from build123d import *

# Parameters (mm, degrees)
SKETCH1_W           = 86
SKETCH1_H           = 57
BOSS_EXTRUDE1_DEPTH = 10
SKETCH2_R           = 2
CUT_EXTRUDE1_DEPTH  = 67.213669284
SKETCH4_W           = 96
SKETCH4_H           = 66
SKETCH4_W_2         = 82
SKETCH4_H_2         = 52
BOSS_EXTRUDE2_DEPTH = 2
SKETCH6_W           = 54
SKETCH6_H           = 5
CUT_EXTRUDE2_DEPTH  = 5
SKETCH7_W           = 43
SKETCH7_H           = 5
CUT_EXTRUDE3_DEPTH  = 5
CHAMFER1_SIZE       = 2
CHAMFER2_SIZE       = 1
CHAMFER3_SIZE       = 1
CHAMFER4_SIZE       = 1
SKETCH9_R           = 3.75
CUT_EXTRUDE4_DEPTH  = 2.7
SKETCH10_W          = 65
SKETCH10_H          = 6
CUT_EXTRUDE5_DEPTH  = 4.5
SKETCH11_W          = 14
SKETCH11_H          = 6
CUT_EXTRUDE6_DEPTH  = 4.5


with BuildPart() as part:
    # Sketch1 → Boss-Extrude1 (new body)
    with BuildSketch(Plane(origin=(0, 0, 0), x_dir=(1, 0, 0), z_dir=(0, 1, 0))):
        with BuildLine():
            Line((48, -33), (48, 33))
            Line((48, 33), (-33, 33))
            Line((-33, 33), (-33, 39.5))
            ThreePointArc((-33, 39.5), (-38, 44.5), (-43, 39.5))
            Line((-43, 39.5), (-43, 33))
            Line((-43, 33), (-48, 33))
            Line((-48, 33), (-48, -33))
            Line((-48, -33), (-38, -33))
            Line((-38, -33), (-38, -39.5))
            ThreePointArc((-38, -39.5), (-33, -44.5), (-28, -39.5))
            Line((-28, -39.5), (-28, -33))
            Line((-28, -33), (28, -33))
            Line((28, -33), (28, -39.5))
            ThreePointArc((28, -39.5), (33, -44.5), (38, -39.5))
            Line((38, -39.5), (38, -33))
            Line((38, -33), (48, -33))
        make_face()
        Rectangle(SKETCH1_W, SKETCH1_H, mode=Mode.SUBTRACT)
    extrude(amount=BOSS_EXTRUDE1_DEPTH)

    # Sketch2 → Cut-Extrude1 (cut, through all)
    with BuildSketch(Plane(origin=(0, 10, 0), x_dir=(1, 0, 0), z_dir=(0, 1, 0))):
        with Locations(Location((-38, 39.5, 0), (0, 0, 270))):
            Circle(SKETCH2_R)
        with Locations(Location((33, -39.5, 0), (0, 0, 270))):
            Circle(SKETCH2_R)
        with Locations(Location((-33, -39.5, 0), (0, 0, 270))):
            Circle(SKETCH2_R)
    extrude(amount=-CUT_EXTRUDE1_DEPTH, mode=Mode.SUBTRACT)

    # Sketch4 → Boss-Extrude2 (add)
    with BuildSketch(Plane(origin=(0, 10, 0), x_dir=(1, 0, 0), z_dir=(0, 1, 0))):
        Rectangle(SKETCH4_W, SKETCH4_H)
        Rectangle(SKETCH4_W_2, SKETCH4_H_2, mode=Mode.SUBTRACT)
    extrude(amount=BOSS_EXTRUDE2_DEPTH)

    # Sketch6 → Cut-Extrude2 (cut)
    with BuildSketch(Plane.ZY.offset(48)):
        with Locations((0, 2.5)):
            Rectangle(SKETCH6_W, SKETCH6_H)
    extrude(amount=-CUT_EXTRUDE2_DEPTH, mode=Mode.SUBTRACT)

    # Sketch7 → Cut-Extrude3 (cut)
    with BuildSketch(Plane(origin=(48, 0, 0), x_dir=(0, 0, -1), z_dir=(1, 0, 0))):
        with Locations((1.5, 2.5)):
            Rectangle(SKETCH7_W, SKETCH7_H)
    extrude(amount=-CUT_EXTRUDE3_DEPTH, mode=Mode.SUBTRACT)

    # Chamfer1
    chamfer1_edges = [part.edges().sort_by_distance(p)[0] for p in [
        (-41, 12, 0),
        (0, 12, 26),
        (41, 12, 0),
        (0, 12, -26),
    ]]
    chamfer(chamfer1_edges, length=CHAMFER1_SIZE - 0.0001)  # a hair under: the kernel refuses the full size

    # Chamfer2
    chamfer2_edges = [part.edges().sort_by_distance(p)[0] for p in [
        (-48, 12, 0),
        (0, 12, 33),
        (48, 12, 0),
        (0, 12, -33),
    ]]
    chamfer(chamfer2_edges, length=CHAMFER2_SIZE)

    # Chamfer3
    chamfer3_edges = [part.edges().sort_by_distance(p)[0] for p in [
        (-48, 5.5, -33),
    ]]
    chamfer(chamfer3_edges, length=CHAMFER3_SIZE)

    # Chamfer4
    chamfer4_edges = [part.edges().sort_by_distance(p)[0] for p in [
        (48, 5.5, 33),
        (-48, 5.5, 33),
        (48, 5.5, -33),
    ]]
    chamfer(chamfer4_edges, length=CHAMFER4_SIZE)

    # Sketch9 → Cut-Extrude4 (cut)
    with BuildSketch(Plane(origin=(0, 10, 0), x_dir=(1, 0, 0), z_dir=(0, 1, 0))):
        with Locations(Location((-38, 39.5, 0), (0, 0, 270))):
            Circle(SKETCH9_R)
        with Locations(Location((-33, -39.5, 0), (0, 0, 270))):
            Circle(SKETCH9_R)
        with Locations(Location((33, -39.5, 0), (0, 0, 270))):
            Circle(SKETCH9_R)
    extrude(amount=-CUT_EXTRUDE4_DEPTH, mode=Mode.SUBTRACT)

    # Sketch10 → Cut-Extrude5 (cut)
    with BuildSketch(Plane(origin=(0, 0, -33), x_dir=(-1, 0, 0), z_dir=(0, 0, -1))):
        with Locations((0.5, 3)):
            Rectangle(SKETCH10_W, SKETCH10_H)
    extrude(amount=-CUT_EXTRUDE5_DEPTH, mode=Mode.SUBTRACT)

    # Sketch11 → Cut-Extrude6 (cut)
    with BuildSketch(Plane.XY.offset(33)):
        with Locations((-21, 3)):
            Rectangle(SKETCH11_W, SKETCH11_H)
    extrude(amount=-CUT_EXTRUDE6_DEPTH, mode=Mode.SUBTRACT)


solid = part.part
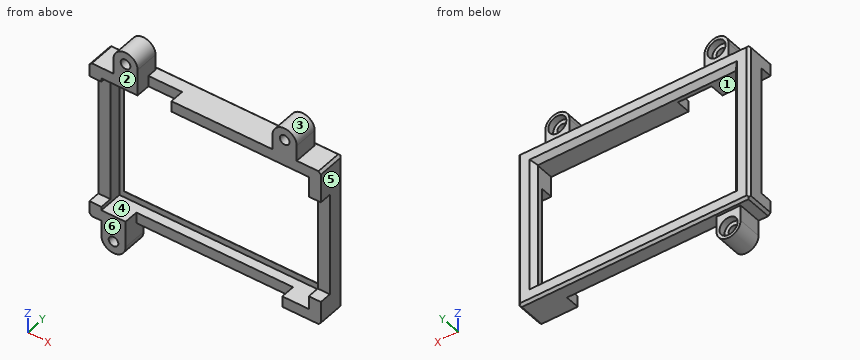
Read the model definition and answer for the solid it produces. Units are mm, in the model's axes. Face numbers are marked on the shaded views. A direction names the side the tool comes from. Round coordinates to 2 decimals unless told otherwise and drop trailing zeros.
1) Straight lines are drawn through the part: L1, parallel to X at y = 5.5, z = 39.5; L2, parallel to X at y = 8.7, z = 39.5; L3, parallel to X at y = 5, z = 35.5. For each, find the intervals that lie inside material, in ascending order.
2) Flat-ended cylindrical pins translate along their axes: pin 1 (8.5 mm diameter, centred on x = -33, z = 39.5, fed in from +Y); pin 2 (5.5 mm diameter, centred on x = 44.5, y = 2.5, fed in from +Z); pin 3 (1.5 mm diameter, centred on x = -46, y = 2.5, fed in from -Z). Find the tip coordinate at first contact, or state that the pin passes through.
3) The mould has two halves that part along X. Classify the marked faces 3, 4, 5 and 6: released by +X, released by -X, zero draft, split by the parting line, or undercut.
4) The part is cut by section C-C on y = 1.5. Give the number of separate pieces and of enclosed holes in the cut face, plus the area to 3 significant figures.
5) For the marked faces 1 and 2, determine the directions among +Z, -Z, +X, -X, +Y, -Y from which every point of the face is accessible in a straight line to the end or side of a thin tool.
Resolved:
1. L1: x = -38 to -35, -31 to -28, 28 to 31, 35 to 38
1. L2: x = -38 to -36.75, -29.25 to -28, 28 to 29.25, 36.75 to 38
1. L3: x = -38 to -28, 28 to 38
2. pin 1: stops at y = 10
2. pin 2: stops at z = 33
2. pin 3: stops at z = -33
3. face 3: undercut
3. face 4: undercut
3. face 5: released by +X
3. face 6: zero draft
4. separate pieces: 4
4. enclosed holes: 3
4. area: 867 mm2
5. face 1: -Y
5. face 2: +Z, -Z, +X, -X, -Y
